For this review, take the finished solid that the model builds, in its own axes (mm). A direction names the side the tool comes from. Coordinates: 2 decimals unless noted, no trailing zeros. Loops run counter-clockwise (first coordinate to the right, second up) from the corner with the lowest first, then second, coordinate; pieces in that order, holes last. Notation, with made-up numbers: (-33, 11.25) - (-17, 11.25) arc R28 ccw to (-17, 47.25) - close; hole circle Ø4 at (79.5, 45). An arc over 180 degrees is marked (long way). One line per item, written item: value. Start each with the question number.
1. To check wall thickness, follow line 1 (Y direction, x = -41, z = -52.5); line 2 (Y direction, x = 28.5, z = -47); line 3 (X direction, y = -10.5, z = -46.5). State the ranges of each line that lie inside material, in increasing order. Write a range as from..to.
2. Take a section at D-D, the plane x = 43. State the section outline as (y, z) points, and give its area (3 significant figures).
3. Take a section at B-B, the plane y = 5.5. Count the separate pieces of the cut face and the enclosed holes in it, and give its area (3 significant figures).
4. Take a section at C-C, the plane x = -23. State the section outline as (y, z) points, and give its area (3 significant figures).
5. Insertion check: pin 1 (0.9 mm diameter, centred on y = -2, z = -53, fed in from +X); pin 2 (4 mm diameter, centred on x = -4.5, y = 18.5, fed in from +Z); pin 3 (0.9 mm diameter, centred on y = -6.5, z = -41, fed in from +X). Each pin has a flat end and moves straight along its axis. Give the tip position at first contact, or say it passes through.
6. Take a section at A-A, the plane x = -41. State the section outline as (y, z) points, and give its area (3 significant figures).
7. The part is to be moulded in two halves that separate along X. For faces 1 (the face through (-37.998, 6.745, -52.521)), 2 (the face through (-1, 23.4, -46)), 3 (the face through (40.5, 0, -53)), 4 (the face through (49.4, -0.3, -52)), say which applies: released by +X, released by -X, zero draft, split by the parting line, or undercut.
8. For faces 5 (the face through (49.9, -0.3, -40.8)), 6 (the face through (51.5, 0, -46)), 7 (the face through (-49.5, -0.3, -51.9)), 8 (the face through (-1, 22, -45)), 9 (the face through (43, -12, -53)), list the 3-axis set-ups (+Z, -Z, +X, -X, +Y, -Y) from which the entire face can be reached by the end or side of a thin tool; tool diameter is ignored.
```python
from build123d import *

# Parameters (mm, degrees)
SKETCH010_W       = 103
SKETCH010_H       = 15
PAD005_DEPTH      = 25
PAD005_DEPTH_BACK = 25
FILLET004_R       = 7
THICKNESS001_T    = -3
SKETCH011_W       = 64
SKETCH011_H       = 40
POCKET002_DEPTH   = 3.001
SKETCH012_W       = 103
SKETCH012_H       = 50
SKETCH012_W_2     = 99.8
SKETCH012_H_2     = 46.8
POCKET003_DEPTH   = 5
SKETCH111_W       = 103
SKETCH111_H       = 1.6
POCKET046_DEPTH   = 10.001
FILLET005_R       = 1.4
FILLET042_R       = 1
SKETCH052_R       = 3.25
SKETCH052_W       = 2
SKETCH052_H       = 24
POCKET021_DEPTH   = 15.001
POCKET_START      = -5
POCKET_DEPTH      = 36.8
POCKET044_START   = -17
POCKET044_DEPTH   = 18
FILLET052_R       = 1.6


with BuildPart() as part:
    # Sketch010 → Pad005 (new body, two sides)
    with BuildSketch(Plane.XZ) as pad005_sk:
        Rectangle(SKETCH010_W, SKETCH010_H)
    extrude(amount=-PAD005_DEPTH)
    extrude(pad005_sk.sketch, amount=PAD005_DEPTH_BACK)

    # Fillet004
    fillet004_edges = [part.edges().sort_by_distance(p)[0] for p in [
        (-51.5, 0, -7.5),
        (51.5, 0, -7.5),
    ]]
    fillet(fillet004_edges, radius=FILLET004_R)

    # Thickness001
    thickness001_openings = [part.faces().sort_by_distance(p)[0] for p in [
        (0, 0, 7.5),
    ]]
    offset(amount=THICKNESS001_T, openings=thickness001_openings)

    # Sketch011 (on Face15 of Thickness001) → Pocket002 (cut, through all)
    with BuildSketch(Plane.XY.offset(-4.5)):
        Rectangle(SKETCH011_W, SKETCH011_H)
    extrude(amount=-POCKET002_DEPTH, mode=Mode.SUBTRACT)

    # Sketch012 (on Face4 of Pocket002) → Pocket003 (cut)
    with BuildSketch(Plane.XY.offset(7.5)):
        Rectangle(SKETCH012_W, SKETCH012_H)
        Rectangle(SKETCH012_W_2, SKETCH012_H_2, mode=Mode.SUBTRACT)
    extrude(amount=-POCKET003_DEPTH, mode=Mode.SUBTRACT)

    # Sketch111 (on Face5 of Pocket003) → Pocket046 (cut, through all)
    with BuildSketch(Plane.XY.offset(2.5)):
        with Locations((0, -24.2)):
            Rectangle(SKETCH111_W, SKETCH111_H)
        with Locations((0, 24.2)):
            Rectangle(SKETCH111_W, SKETCH111_H)
    extrude(amount=-POCKET046_DEPTH, mode=Mode.SUBTRACT)

    # Fillet005
    fillet005_edges = [part.edges().sort_by_distance(p)[0] for p in [
        (-51.5, 0, -0.5),
        (0, -23.4, -7.5),
        (-44.5, 0, -7.5),
        (0, 23.4, -7.5),
    ]]
    fillet(fillet005_edges, radius=FILLET005_R)

    # Fillet042
    fillet042_edges = [part.edges().sort_by_distance(p)[0] for p in [
        (0, 23.4, 7.5),
        (49.9, 0, 7.5),
        (-49.9, 0, 7.5),
        (-49.9, 0, 2.5),
        (49.9, 0, 2.5),
        (0, -23.4, 7.5),
    ]]
    fillet(fillet042_edges, radius=FILLET042_R)

    # Sketch052 (on Face20 of Fillet005) → Pocket021 (cut, through all)
    with BuildSketch(Plane(origin=(0, 0, -7.5), x_dir=(1, 0, 0), z_dir=(0, 0, -1))):
        with Locations((-41, -5.5)):
            Circle(SKETCH052_R)
        with Locations((36, 0)):
            Rectangle(SKETCH052_W, SKETCH052_H)
        with Locations((39.5, 0)):
            Rectangle(SKETCH052_W, SKETCH052_H)
        with Locations((43, 0)):
            Rectangle(SKETCH052_W, SKETCH052_H)
    extrude(amount=-POCKET021_DEPTH, mode=Mode.SUBTRACT)

    # Sketch013 (on Face10 of Pocket003) → Pocket (cut)
    with BuildSketch(Plane.XZ.offset(23.4).offset(POCKET_START)):
        Polygon((49.9, 5.55), (49.9, 4.45), (49.15, 5.55), align=None)
        Polygon((-49.15, 5.55), (-49.9, 5.55), (-49.9, 4.45), align=None)
    extrude(amount=-POCKET_DEPTH, mode=Mode.SUBTRACT)

    # Sketch014 (on Face8 of Fillet042) → Pocket044 (cut)
    with BuildSketch(Plane.YZ.offset(49.9).offset(POCKET044_START)):
        Polygon((23.4, 5.55), (23.4, 4.45), (22.65, 5.55), align=None)
        Polygon((-23.4, 5.55), (-23.4, 4.45), (-22.65, 5.55), align=None)
    pocket044 = extrude(amount=-POCKET044_DEPTH, mode=Mode.SUBTRACT)

    # Mirrored011: Pocket044 across YZ
    add(pocket044.mirror(Plane.YZ), mode=Mode.SUBTRACT)

    # Fillet052
    fillet052_edges = [part.edges().sort_by_distance(p)[0] for p in [
        (-32, 0, -4.5),
        (0, 20, -4.5),
        (32, 0, -4.5),
        (0, -20, -4.5),
    ]]
    fillet(fillet052_edges, radius=FILLET052_R)


with BuildPart() as part_1:
    # Body002 placement: moved
    add(part.part.moved(Location((0, 0, -46.5))))


solid = part_1.part
```
Solutions:
1. line 1: -23.4..2.25, 8.75..23.4
1. line 2: -23.4..-22, 22..23.4
1. line 3: -51.5..-48.5, 48.5..51.5
2. outline: (-23.4, -52.6) arc R1.4 ccw to (-22, -54) - (-12, -54) - (-12, -51) - (-22, -51) - (-22, -39) - (-22.4, -39) arc R1 ccw to (-23.4, -40) - close; (12, -54) - (22, -54) arc R1.4 ccw to (23.4, -52.6) - (23.4, -40) arc R1 ccw to (22.4, -39) - (22, -39) - (22, -51) - (12, -51) - close
2. area: 101 mm2
3. separate pieces: 6
3. enclosed holes: 0
3. area: 119 mm2
4. outline: (-23.4, -52.6) arc R1.4 ccw to (-22, -54) - (-20, -54) - (-20, -52.6) arc R1.6 ccw to (-21.6, -51) - (-22, -51) - (-22, -39) - (-22.4, -39) arc R1 ccw to (-23.4, -40) - (-23.4, -40.95) - (-22.65, -40.95) - (-23.4, -42.05) - close; (20, -54) - (22, -54) arc R1.4 ccw to (23.4, -52.6) - (23.4, -42.05) - (22.65, -40.95) - (23.4, -40.95) - (23.4, -40) arc R1 ccw to (22.4, -39) - (22, -39) - (22, -51) - (21.6, -51) arc R1.6 ccw to (20, -52.6) - close
4. area: 50.8 mm2
5. pin 1: x = 48.77
5. pin 2: z = -51.44
5. pin 3: x = 49.9
6. outline: (-23.4, -52.6) arc R1.4 ccw to (-22, -54) - (2.25, -54) - (2.25, -51) - (-22, -51) - (-22, -39) - (-22.4, -39) arc R1 ccw to (-23.4, -40) - close; (8.75, -54) - (22, -54) arc R1.4 ccw to (23.4, -52.6) - (23.4, -40) arc R1 ccw to (22.4, -39) - (22, -39) - (22, -51) - (8.75, -51) - close
6. area: 153 mm2
7. face 1: undercut
7. face 2: zero draft
7. face 3: undercut
7. face 4: released by +X
8. face 5: +Z, +X, +Y, -Y
8. face 6: +Z, -Z, +X, +Y, -Y
8. face 7: -Z, -X, +Y, -Y
8. face 8: +Z
8. face 9: +Z, -Z
